```python
from build123d import *
from build123d.topology import SkipClean

# Parameters (mm, degrees)
CUT_EXTRUDE1_DEPTH = 0.966
CIRPATTERN1_COUNT  = 6


with BuildPart() as part:
    # Sketch2 → Revolve1 (revolve)
    with BuildSketch(Plane(origin=(0, 0, 0), x_dir=(0, 0, -1), z_dir=(1, 0, 0))):
        Polygon((1.38, 1.25), (6.0425, 1.25), (6.38, 0.9125), (6.38, 0), (1.38, 0), align=None)
    revolve(axis=Axis((0, 0, -6.38), (0, 0, 1)))


with BuildPart() as body_2:
    # Sketch3 → Revolve2 (revolve)
    with BuildSketch(Plane(origin=(0, 0, 0), x_dir=(0, 0, -1), z_dir=(1, 0, 0)), mode=Mode.PRIVATE) as revolve2_sk:
        with BuildLine():
            Line((1.38, 0), (1.38, 2.375))
            Line((1.38, 2.375), (1.173, 2.375))
            ThreePointArc((1.173, 2.375), (0.500332222, 1.917105021), (0, 1.275375))
            Line((0, 1.275375), (0, 0))
            Line((0, 0), (1.38, 0))
        make_face()
    revolve(revolve2_sk.sketch.rotate(Axis((0, 0, 0), (0, 0, -1)), 90), axis=Axis((0, 0, 0), (0, 0, -1)))

    # Combine1: union part
    add(part.part)

    # Sketch4 → Cut-Extrude1 (cut)
    with BuildSketch(Plane.XY):
        with BuildLine():
            Line((0, 0), (-0.898826116, 0.5189375))
            ThreePointArc((-0.898826116, 0.5189375), (-0.910259221, 0.475549675), (-0.89810803, 0.432357455))
            ThreePointArc((-0.89810803, 0.432357455), (-0.77840625, 0), (-0.89810803, -0.432357455))
            ThreePointArc((-0.89810803, -0.432357455), (-0.910259221, -0.475549675), (-0.898826116, -0.5189375))
            Line((-0.898826116, -0.5189375), (0, 0))
        make_face()
    cut_extrude1 = extrude(amount=-CUT_EXTRUDE1_DEPTH, mode=Mode.SUBTRACT)

    # CirPattern1: Cut-Extrude1 ×6 about axis
    cirpattern1_axis = Axis((0, 0, 0), (0, 0, 1))
    for i in range(1, CIRPATTERN1_COUNT):
        add(cut_extrude1.rotate(cirpattern1_axis, i * 360 / CIRPATTERN1_COUNT), mode=Mode.SUBTRACT)

    # Sketch5 → Cut-Revolve1 (revolve, cut)
    with SkipClean():  # the faces are left unmerged after this step: merging them gives an invalid solid
        with BuildSketch(Plane(origin=(0, 0, 0), x_dir=(0, 0, -1), z_dir=(1, 0, 0))):
            with BuildLine():
                Line((-1.767310001, 2.089310001), (-1.767310001, -2.089310001))
                ThreePointArc((-1.767310001, -2.089310001), (0.322, 0), (-1.767310001, 2.089310001))
            make_face()
        revolve(axis=Axis((0, 2.089310001, 1.767310001), (0, -1, 0)), mode=Mode.SUBTRACT)


solid = body_2.part
```
Work out the finished part from the listing and answer in its coordinate system (mm). A direction names the side the tool comes from. Give positions to 0.01 mm unless a question says otherwise; leave off trailing zeros. Loops run counter-clockwise (first coordinate to the right, second up) from the corner with the lowest first, then second, coordinate; pieces in that order, holes last. Notation, with made-up numbers: (-2, 65) - (34, 65) arc R32 ccw to (34, 98) - close; hole circle Ø1 at (64, -9.5). An arc over 180 degrees is marked (long way). Use CSV: the item, a comma, the result in double quotes. Start each with the question number.
(1) Find section D-D, the plane x = 2. Determine the outline of the cut face in (y, z), plus the area to 3 significant figures.
(2) This flat-tipped pin is pushed along its axis until it touches: pin 1 (1.5 mm diameter, centred on x = -1, z = -5, fed in from +Y). Where does it stop, or does it pass through?
(3) Find section A-A, the plane z = -0.25. Determine the outline of the cut face in (x, y).
(4) Find section C-C, the plane y = 1.45. Determine the outline of the cut face in (x, z), plus the area to 3 significant figures.
(5) Find section B-B, the plane z = -2. Determine the outline of the cut face in (x, y), plus the area to 3 significant figures.
(6) Determine the mould class of faces 1 (the face through (0.78, -0.01, -0.51)), 2 (the face through (-1, 1, -1.38)), 3 (the face through (1.22, -0.27, -3.74)) for opening direction Y: released by +Y, released by -Y, zero draft, split by the parting line, or undercut.
(7) A tool of negligible diameter and unlimited length cuts with its end or side. For faces 4 (the face through (-0.78, 0.01, -0.51)), 5 (the face through (0, 0, -6.38)), from which of +Z, -Z, +X, -X, +Y, -Y can it reach the whole face along a straight path? Write none if from no direction.
(8) Find the intervals of material crossed by L1, parallel to X at y = 0.75, z = -0.75; L2, parallel to Z at x = -0.35, y = 0.45, in increasing order.
Results found:
1,outline,"(-1.28, -1.38) - (1.28, -1.38) - (1.28, -1.17) arc R1.7 ccw to (-1.28, -1.17) - close"
1,area,"1.56 mm^2"
2,pin 1,"y = 1.22"
3,outline,"circle Ø3.29 at (0, 0); hole (-0.9, -0.43) arc R0.09 ccw to (-0.82, -0.56) arc R0.84 cw to (-0.07, -0.99) arc R0.09 ccw to (0.07, -0.99) arc R0.84 cw to (0.82, -0.56) arc R0.09 ccw to (0.9, -0.43) arc R0.84 cw to (0.9, 0.43) arc R0.09 ccw to (0.82, 0.56) arc R0.84 cw to (0.07, 0.99) arc R0.09 ccw to (-0.07, 0.99) arc R0.84 cw to (-0.82, 0.56) arc R0.09 ccw to (-0.9, 0.43) arc R0.84 cw to start"
4,outline,"(-1.88, -1.38) - (1.88, -1.38) - (1.88, -1.17) arc R2.19 ccw to (-1.88, -1.17) - close"
4,area,"3.62 mm^2"
5,outline,"circle Ø2.5 at (0, 0)"
5,area,"4.91 mm^2"
6,face 1,"undercut"
6,face 2,"zero draft"
6,face 3,"split by the parting line"
7,face 4,"+Z"
7,face 5,"-Z, +X, -X, +Y, -Y"
8,L1,"-1.99 to -0.28, 0.28 to 1.99"
8,L2,"-6.38 to -0.97"
